Verification items for this drawing (mm, ordinates from the low corner). A direction names the side the tool comes from. Give positions to 0.01 mm unless a question says otherwise; leave off trailing zeros. Order: outer loops, then holes, each group sorted by start corner. A loop starts at its lowest first (then second) coordinate and runs counter-clockwise, first axis right, second up.
(1) Gauge pin test, flat ends, axial feed: pin 1 (1.5 mm diameter, centred on y = 1, z = 7.5, fed in from +X); pin 2 (2 mm diameter, centred on x = 4.5, z = 3.5, fed in from -Y). Record the tip position at first contact, or that the pin passes through.
(2) Sectioned sample at B-B on y = 7.75. Record the cut outline in (x, z), plus the area to 3 significant figures.
(3) Sectioned sample at A-A on z = 6.5. Record the cut outline in (x, y) (3 decimals).
(4) Sectioned sample at C-C on z = 7.5. Record the cut outline in (x, y) (1 decimal), plus the area to 3 significant figures.
(5) Scan lines: L1, parallel to Z at x = 3.5, y = 7; L2, parallel to Y at x = 2.65, z = 6.5; L3, parallel to Z at x = 2.4, y = 4.75. Record each from-to range of solid material in increasing order.
(6) Access from +Z, -Z, +X, -X, +Y, -Y to the whole of each face (thin tool, end or side, straight path). Record for the marked faces 1 and 2.
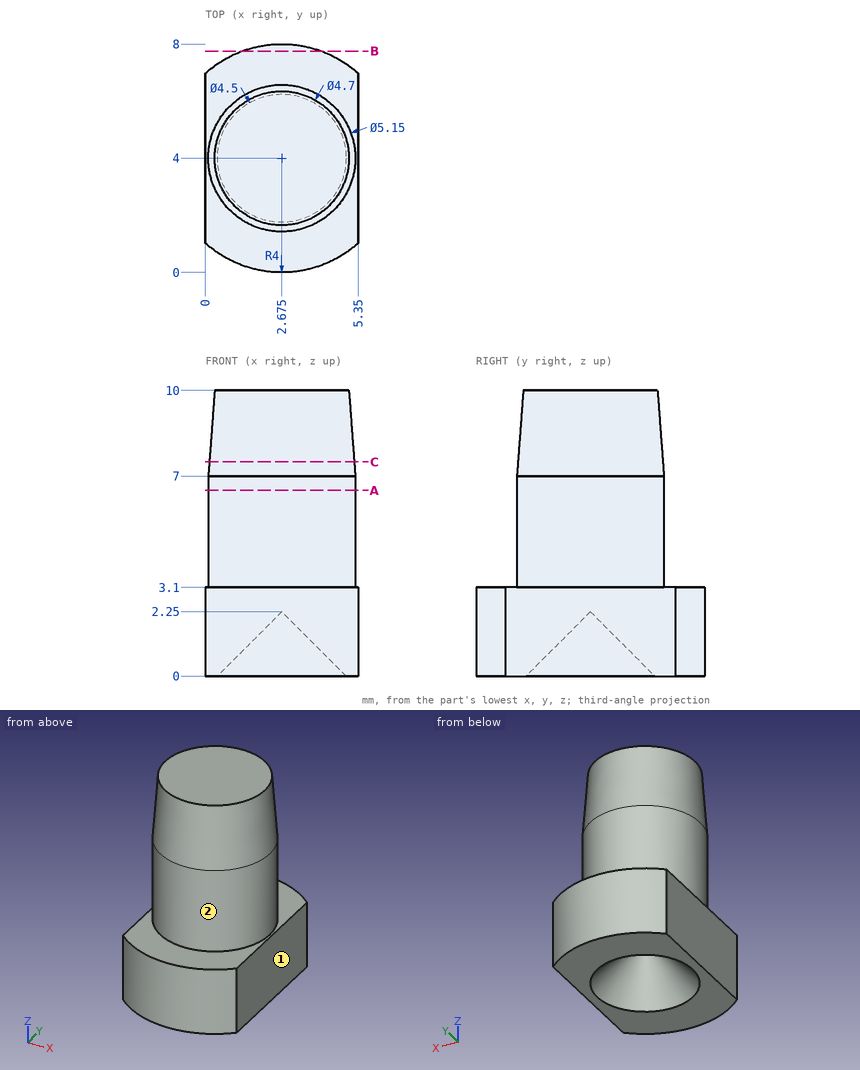
Ans:
1. pin 1: stops at x = 3.85
1. pin 2: stops at y = 0.1
2. outline: (1.28, 0) - (4.07, 0) - (4.07, 3.1) - (1.28, 3.1) - close
2. area: 8.63 mm2
3. outline: circle Ø5.15 at (2.675, 4)
4. outline: circle Ø5.1 at (2.7, 4)
4. area: 20.2 mm2
5. L1: z = 0 to 3.1
5. L2: y = 1.43 to 6.57
5. L3: z = 1.45 to 10
6. face 1: +Z, -Z, +X, +Y, -Y
6. face 2: +Z
